from build123d import *

# Parameters (mm, degrees)
SKETCH1_R           = 14
BOSS_EXTRUDE1_DEPTH = 4
SKETCH2_R           = 14
SKETCH2_R_2         = 12
BOSS_EXTRUDE2_DEPTH = 2
SKETCH3_R           = 1
CUT_EXTRUDE1_DEPTH  = 21.199009877
SKETCH4_R           = 1.75
CUT_EXTRUDE2_DEPTH  = 21.199009877
SKETCH5_R           = 1
BOSS_EXTRUDE3_DEPTH = 1


with BuildPart() as part:
    # Sketch1 → Boss-Extrude1 (new body)
    with BuildSketch(Plane.XY):
        Circle(SKETCH1_R)
    extrude(amount=BOSS_EXTRUDE1_DEPTH)

    # Sketch2 → Boss-Extrude2 (add)
    with BuildSketch(Plane.XY.offset(4)):
        Circle(SKETCH2_R)
        Circle(SKETCH2_R_2, mode=Mode.SUBTRACT)
    extrude(amount=BOSS_EXTRUDE2_DEPTH)

    # Sketch3 → Cut-Extrude1 (cut, through all)
    with BuildSketch(Plane.XY.offset(4)):
        with Locations((0, 8)):
            Circle(SKETCH3_R)
        with Locations((8, 0)):
            Circle(SKETCH3_R)
        with Locations((0, -8)):
            Circle(SKETCH3_R)
        with Locations((-8, 0)):
            Circle(SKETCH3_R)
    extrude(amount=-CUT_EXTRUDE1_DEPTH, mode=Mode.SUBTRACT)

    # Sketch4 → Cut-Extrude2 (cut, through all)
    with BuildSketch(Plane.XY.offset(4)):
        with Locations((0, 4.75)):
            Circle(SKETCH4_R)
        with Locations((0, -4.75)):
            Circle(SKETCH4_R)
    extrude(amount=-CUT_EXTRUDE2_DEPTH, mode=Mode.SUBTRACT)

    # Sketch5 → Boss-Extrude3 (add)
    with BuildSketch(Plane.XY.offset(4)):
        with Locations((-6.320770843, -6.320770843)):
            Circle(SKETCH5_R)
        with Locations((-6.320770843, 6.320770843)):
            Circle(SKETCH5_R)
        with Locations((6.320770843, 6.320770843)):
            Circle(SKETCH5_R)
        with Locations((6.320770843, -6.320770843)):
            Circle(SKETCH5_R)
    extrude(amount=BOSS_EXTRUDE3_DEPTH)


solid = part.part
The listing builds one solid part. Answer for the finished solid, in the listing's coordinates (mm). A direction names the side the tool comes from. Coordinates: 2 decimals unless noted, no trailing zeros. Write each loop counter-clockwise with the first axis right and the second up, starting at its lowest first coordinate (ties: lowest second). Pieces come first, ordered by that corner, then holes. Notation, with made-up numbers: (71, -6) - (91, -6) arc R19 cw to (91, 6) - close; hole circle Ø7 at (22, 7). An arc over 180 degrees is marked (long way). Return JSON: item names as keys, results as strings.
1. Each of these flat-tipped pins is pushed along its axis until it touches: pin 1 Ø2 at (x, z) = (10.5, 5) entering from -Y; pin 2 Ø6 at (x, y) = (6.5, 5.5) entering from +Z; pin 3 Ø1.5 at (x, z) = (1, 1) entering from +Y; pin 4 Ø2 at (x, y) = (0, 4.75) entering from -Z. Where does it stop, or does it pass through?
Final values:
{"pin 1": "y = -10.28", "pin 2": "z = 5", "pin 3": "y = 14", "pin 4": "through"}
2. For a pull along Y with two mould halves and no side action, classify faces 3 (the face through (6.104, 5.345, 4.493)), 4 (the face through (12.932, -5.362, 2.958)), 5 (the face through (0, 0, 0)), 6 (the face through (-7.114, 5.712, 4.493)) as +Y half, -Y half, draft (parallel to the pull), parting line (faces both ways), or undercut.
Final values:
{"face 3": "undercut", "face 4": "parting line", "face 5": "draft", "face 6": "undercut"}
3. The part is cut by section C-C on x = 8.5. Determine the outline of the cut face in (y, z).
Final values:
{"outline": "(-11.12, 0) - (-0.87, 0) - (-0.87, 4) - (-8.47, 4) - (-8.47, 6) - (-11.12, 6) - close; (0.87, 0) - (11.12, 0) - (11.12, 6) - (8.47, 6) - (8.47, 4) - (0.87, 4) - close"}
4. Consider line 1 along Y through (x, z) = (0, 1.4); line 2 along Y through (x, z) = (0, 4.9); line 3 along Z through (x, y) = (0, 2.25). Determine where each line is inside the solid, lowest interval first.
Final values:
{"line 1": "-14 to -9, -7 to -6.5, -3 to 3, 6.5 to 7, 9 to 14", "line 2": "-14 to -12, 12 to 14", "line 3": "0 to 4"}
5. The part is cut by section D-D on x = 0. Determine the outline of the cut face in (y, z).
Final values:
{"outline": "(-14, 0) - (-9, 0) - (-9, 4) - (-12, 4) - (-12, 6) - (-14, 6) - close; (-7, 0) - (-6.5, 0) - (-6.5, 4) - (-7, 4) - close; (-3, 0) - (3, 0) - (3, 4) - (-3, 4) - close; (6.5, 0) - (7, 0) - (7, 4) - (6.5, 4) - close; (9, 0) - (14, 0) - (14, 6) - (12, 6) - (12, 4) - (9, 4) - close"}
6. The part is cut by section B-B on z = 1.2. Determine the outline of the cut face in (x, y), then the cut area to 3 significant figures.
Final values:
{"outline": "circle Ø28 at (0, 0); hole circle Ø2 at (-8, 0); hole circle Ø3.5 at (0, -4.75); hole circle Ø3.5 at (0, 4.75); hole circle Ø2 at (0, -8); hole circle Ø2 at (0, 8); hole circle Ø2 at (8, 0)", "area": "584 mm^2"}
7. Which of the six approach directions +Z, -Z, +X, -X, +Y, -Y give full straight-line access (tool end or side, diameter ignored) to faces 1 (the face through (0, 9, 2)), 2 (the face through (-11.99, 0.53, 4.99))?
Final values:
{"face 1": "+Z, -Z", "face 2": "+Z"}
8. The part is cut by section A-A on y = 0. Determine the outline of the cut face in (x, z), then the cut area to 3 significant figures.
Final values:
{"outline": "(-14, 0) - (-9, 0) - (-9, 4) - (-12, 4) - (-12, 6) - (-14, 6) - close; (-7, 0) - (7, 0) - (7, 4) - (-7, 4) - close; (9, 0) - (14, 0) - (14, 6) - (12, 6) - (12, 4) - (9, 4) - close", "area": "104 mm^2"}
